Here's how the part is built. I have some questions about the finished solid (model axes, mm). Face numbers are marked on the shaded views. A direction names the side the tool comes from. Give positions to 0.01 mm unless a question says otherwise; leave off trailing zeros. Write each loop counter-clockwise with the first axis right and the second up, starting at its lowest first coordinate (ties: lowest second). Pieces come first, ordered by that corner, then holes. Notation, with made-up numbers: (-25, -14) -> (-9, -14) arc R18 ccw to (-9, 21) -> close; hole circle Ø11 at (46.5, 42). An arc over 180 degrees is marked (long way). Use CSV: the item, a comma, the result in double quotes. Start each with the question number.
(1) I need wall thicknesses on L1, parallel to Y at x = 3.25, z = -5.75; L2, parallel to Y at x = -7.25, z = 2; L3, parallel to Z at x = -5.5, y = -1.25. Which ranges of each line are inside material? Lowest first, please. Write a range as [from, to].
(2) If we mould it in two halves opening along Z, with no side actions, what happens to the marked faces 4, 5 and 6? For each: pulls with the +Z half, pulls with the -Z half, needs draft (parallel to the pull), parting line crosses it, or undercut.
(3) For pin 1 Ø0.9 at (y, z) = (-14.5, -0.5) entering from -X; pin 2 Ø3 at (y, z) = (-2.5, 3) entering from +X; pin 3 Ø2.5 at (x, z) = (0, -1) entering from -Y, each with a flat end and sliding along its axis, tell me the tip position at first contact or that it passes through.
(4) Which directions (+Z, -Z, +X, -X, +Y, -Y) give clear straight access to the entire face, cutting with the end or side of a thin tool? Please do the marked faces 1, 2 and 3.
(5) Suppose I cut it at D-D on y = -7.25. List the corners of the cut face in (x, z) for me.
(6) Suppose I cut it at A-A on y = -14.5. List the corners of the cut face in (x, z) for me.
(7) Suppose I cut it at B-B on z = -3.25. Give the number of separate pieces and of enclosed holes in the cut face, plus the area to 3 significant figures.
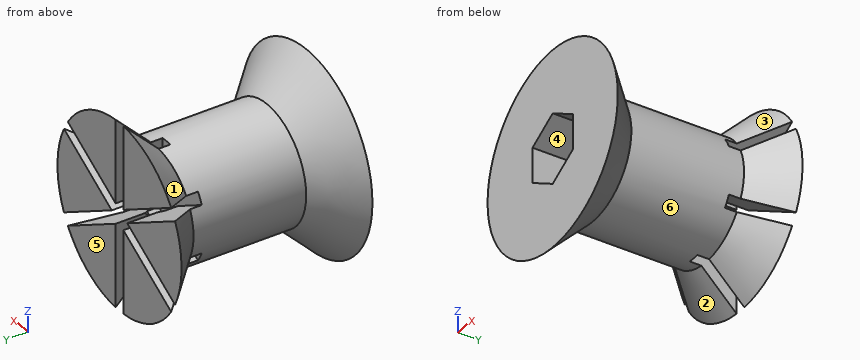
from build123d import *

# Parameters (mm, degrees)
SKETCH_2_R               = 10
EXTRUDE_1_DEPTH          = 3.4
SKETCH_5_W               = 5
SKETCH_5_H               = 8.6
CUT_EXTRUDE_1_DEPTH      = 0.5
PATTERN_CIRCULAR_1_COUNT = 6


with BuildPart() as part:
    # 草图2 → 凸台-拉伸1 (new body)
    with BuildSketch(Plane(origin=(0, -16, 0), x_dir=(-1, 0, 0), z_dir=(0, -1, 0))):
        Circle(SKETCH_2_R)
        Polygon((0, 3.0022214), (-2.6, 1.5011107), (-2.6, -1.5011107), (0, -3.0022214), (2.6, -1.5011107), (2.6, 1.5011107), align=None, mode=Mode.SUBTRACT)
    extrude(amount=-EXTRUDE_1_DEPTH)

    # 草图5 → 旋转1 (revolve)
    with BuildSketch(Plane.XY):
        with Locations((-2.5, -8.3)):
            Rectangle(SKETCH_5_W, SKETCH_5_H)
    revolve(axis=Axis((0, 22.928075319, 0), (0, -1, 0)))

    # 草图6 → 切除-旋转1 (revolve, cut)
    with BuildSketch(Plane.XY):
        Polygon((-5, -12.6), (-10, -17.6), (-10, -12.6), align=None)
    revolve(axis=Axis((0, 0, 0), (0, -1, 0)), mode=Mode.SUBTRACT)

    # 草图7 → 旋转2 (revolve)
    with BuildSketch(Plane.XY):
        Polygon((-5, -4), (0, -4), (0, 0), (-8, 0), (-5, -3), align=None)
    revolve(axis=Axis((0, 2.901504441, 0), (0, -1, 0)))

    # 草图8 → 切除-拉伸1 (cut, symmetric)
    with BuildSketch(Plane(origin=(0, 0, 0), x_dir=(0, 0, -1), z_dir=(1, 0, 0))):
        Polygon((-5, -3), (-8, 0), (0, 0), (0, -4), (-5, -4), align=None)
    cut_extrude_1 = extrude(amount=CUT_EXTRUDE_1_DEPTH, both=True, mode=Mode.SUBTRACT)

    # 阵列(圆周)1: 切除-拉伸1 ×6 about axis
    pattern_circular_1_axis = Axis((0, 0, 0), (0, 1, 0))
    for i in range(1, PATTERN_CIRCULAR_1_COUNT):
        add(cut_extrude_1.rotate(pattern_circular_1_axis, i * 360 / PATTERN_CIRCULAR_1_COUNT), mode=Mode.SUBTRACT)

    # 草图9 → 切除-旋转3 (revolve, cut)
    with BuildSketch(Plane.XY):
        Polygon((0, -4), (-1.5, -4), (-1.5, -3), (0, -1.5), align=None)
    revolve(axis=Axis((0, 4.48946261, 0), (0, -1, 0)), mode=Mode.SUBTRACT)


solid = part.part
Geometry says:
1,L1,"[-16, -14.2], [-1.4, 0]"
1,L2,"[-16, -15.12], [-0.48, 0]"
1,L3,"[-3.91, -3.75], [-2.6, 2.6], [3.75, 3.91]"
2,face 4,"undercut"
2,face 5,"needs draft"
2,face 6,"parting line crosses it"
3,pin 1,"x = -7.33"
3,pin 2,"x = 6.45"
3,pin 3,"y = -12.6"
4,face 1,"+Z, -X"
4,face 2,"-Z, -X"
4,face 3,"+Z, +X"
5,outline,"circle Ø10 at (0, 0)"
6,outline,"circle Ø13.8 at (0, 0); hole (-2.6, -1.5) -> (0, -3) -> (2.6, -1.5) -> (2.6, 1.5) -> (0, 3) -> (-2.6, 1.5) -> close"
7,separate pieces,"3"
7,enclosed holes,"0"
7,area,"136 mm²"
